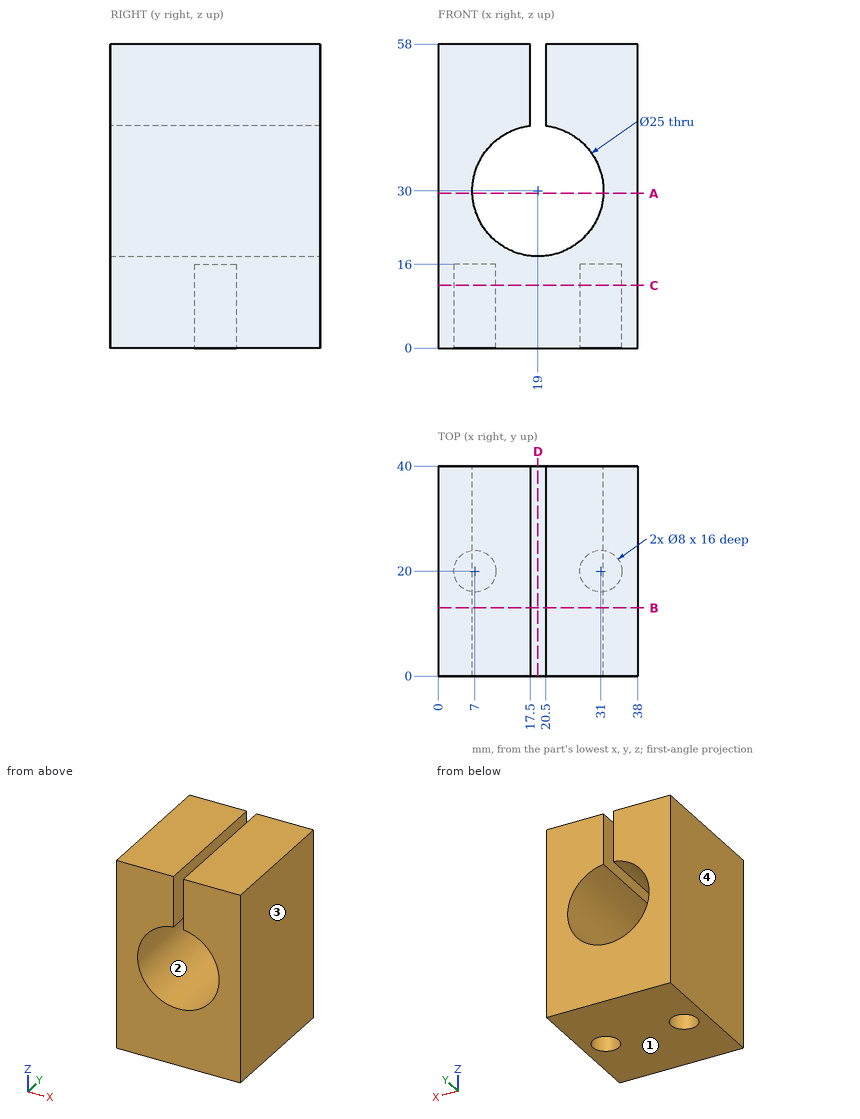
Geometry: see drawing. Coordinates: mm, zero at the bounding-box minimum. Round coordinates to 2 decimals unless told otherwise and drop trailing zeros. Write each loop counter-clockwise with the first axis right and the second up, starting at its lowest first coordinate (ties: lowest second). Pieces come first, ordered by that corner, then holes.
1) Ray query, L1, parallel to X at y = 20, z = 12.25; L2, parallel to Y at x = 7, z = 7; L3, parallel to X at y = 21, z = 30. Return the intervals inside material, ascending.
2) Draft query along X for the marked faces 1, 2, 3 and 4. Return one class per face: pulls with the +X half, pulls with the -X half, needs draft (parallel to the pull), parting line crosses it, or undercut.
3) Contact query for flat-ended pins moving along their axis: P1, Ø5, axis at x = 9, z = 46.5, coming from the -Y side; P2, Ø5, axis at x = 7, y = 20, coming from the -Z side. Output: stop coordinate, or through.
4) Cut plane A-A (z = 29.5). Return the cut outline in (x, y), then the cut area to 3 significant figures.
5) Cut plane B-B (y = 13). Return the cut outline in (x, z).
6) Cut plane C-C (z = 12). Return the cut outline in (x, y).
7) Cut plane D-D (x = 19). Return the cut outline in (y, z).
Geometry says:
1. L1: x = 0 to 3, 11 to 27, 35 to 38
1. L2: y = 0 to 16, 24 to 40
1. L3: x = 0 to 6.5, 31.5 to 38
2. face 1: needs draft
2. face 2: undercut
2. face 3: pulls with the +X half
2. face 4: pulls with the -X half
3. P1: stops at y = 0
3. P2: stops at z = 16
4. outline: (0, 0) - (6.51, 0) - (6.51, 40) - (0, 40) - close; (31.49, 0) - (38, 0) - (38, 40) - (31.49, 40) - close
4. area: 521 mm2
5. outline: (0, 0) - (38, 0) - (38, 58) - (20.5, 58) - (20.5, 42.41) arc R12.5 cw (long way) to (17.5, 42.41) - (17.5, 58) - (0, 58) - close
6. outline: (0, 0) - (38, 0) - (38, 40) - (0, 40) - close; hole circle Ø8 at (7, 20); hole circle Ø8 at (31, 20)
7. outline: (0, 0) - (40, 0) - (40, 17.5) - (0, 17.5) - close
